Autodesk Inventor part; units mm, degrees
ref_plane "YZ Plane" through (0, 0, 0) normal (1, 0, 0) x (0, 1, 0)
ref_plane "XZ Plane" through (0, 0, 0) normal (0, 1, 0) x (-1, 0, 0)
ref_plane "XY Plane" through (0, 0, 0) normal (0, 0, 1) x (1, 0, 0)
sketch "Эскиз1" plane through (0, 0, 0) normal (0, 1, 0) x (-1, 0, 0)
  line L0 (0, 0) -> (49, 0)
  line L1 (49, 0) -> (49, 43)
  line L2 (49, 43) -> (0, 43)
  line L3 (0, 43) -> (0, 0)
  dimension "d0" = 49
  dimension "d1" = 43
extrude "Выдавливание1" add sketch "Эскиз1" along normal blind 1.5
sketch "Эскиз2" plane through (0, 1.5, 0) normal (0, 1, 0) x (1, 0, 0)
  circle A0 centre (-43.5, -4.7) radius 1.5
  circle A1 centre (-43.5, -38.3) radius 1.5
  circle A2 centre (-5.5, -4.7) radius 1.5
  circle A3 centre (-5.5, -38.3) radius 1.5
  line L0 (-49, 0) -> (-49, -43)
  line L1 (0, 0) -> (-49, 0)
  line L2 (-49, -43) -> (0, -43)
  line L3 (0, -43) -> (0, 0)
  dimension "d4" = 3
  dimension "d5" = 3
  dimension "d6" = 3
  dimension "d7" = 3
  dimension "d8" = 5.5
  dimension "d9" = 5.5
  dimension "d10" = 4.7
  dimension "d11" = 4.7
  dimension "d12" = 5.5
  dimension "d13" = 5.5
  dimension "d14" = 4.7
  dimension "d15" = 4.7
extrude "Выдавливание2" cut sketch "Эскиз2" against normal blind 1.5 contours A0 | A1 | A2 | A3
sketch "Эскиз3" plane through (0, 1.5, 0) normal (0, 1, 0) x (1, 0, 0)
  line L0 (0, 0) -> (-49, 0)
  line L1 (-22.5, 0) -> (-12, 0)
  line L2 (-12, 0) -> (-12, -8)
  line L3 (-12, -8) -> (-22.5, -8)
  line L4 (-22.5, -8) -> (-22.5, 0)
  line L5 (0, -43) -> (0, 0)
  line L6 (-49, -43) -> (0, -43)
  line L7 (-22.5, -43) -> (-12, -43)
  line L8 (-12, -43) -> (-12, -35)
  line L9 (-12, -35) -> (-22.5, -35)
  line L10 (-22.5, -35) -> (-22.5, -43)
  line L11 (0, -33) -> (-8, -33)
  line L12 (-8, -33) -> (-8, -10)
  line L13 (-8, -10) -> (0, -10)
  line L14 (0, -10) -> (0, -33)
  point P0 (0, -10)
  dimension "d18" = 10.5
  dimension "d19" = 8
  dimension "d20" = 12
  dimension "d21" = 8
  dimension "d22" = 8
  dimension "d23" = 10
  dimension "d24" = 10
extrude "Выдавливание3" add sketch "Эскиз3" along normal blind 11
chamfer "Фаска1" distance 3 angle 45 3 edges at (-17.25, 12.5, 8) (-17.25, 12.5, 35) (-8, 12.5, 21.5)
fillet "Сопряжение1" radius 3 4 edges at (0, 0.75, 0) (0, 0.75, 43) (-49, 0.75, 43) (-49, 0.75, 0)
sketch "Эскиз4" plane through (0, 1.5, 0) normal (0, 1, 0) x (1, 0, 0)
  line L0 (-49, -3) -> (-49, -40)
  line L1 (-49, -33) -> (-33, -33)
  line L2 (-33, -33) -> (-33, -10)
  line L3 (-33, -10) -> (-49, -10)
  line L4 (-49, -10) -> (-49, -33)
  line L5 (-22.5, 0) -> (-46, 0)
  line L6 (-46, -43) -> (-22.5, -43)
  point P0 (0, 0)
  dimension "d31" = 23
  dimension "d32" = 16
  dimension "d33" = 43
  dimension "d34" = 10
extrude "Выдавливание4" add sketch "Эскиз4" along normal blind 25
equation "\"d9\" = d8"
equation "\"d11\" = d10"
equation "\"d12\" = d8"
equation "\"d13\" = d12"
equation "\"d14\" = d11"
equation "\"d15\" = d11"
equation "\"d21\" = d19"
properties part number "драйвер"
Source: CAD feature listing. Evaluate the final solid. Frame: model axes, mm. A direction names the side the tool comes from. Give positions to 0.01 mm unless a question says otherwise; leave off trailing zeros. Loops run counter-clockwise (first coordinate to the right, second up) from the corner with the lowest first, then second, coordinate; pieces in that order, holes last. Notation, with made-up numbers: (17, 63.5) -> (36, 63.5) arc R34 cw to (36, 101.5) -> close; hole circle Ø10 at (43, -28.5). An arc over 180 degrees is marked (long way). Put each result on its own line as item: value. Start each with the question number.
1) Contact query for flat-ended pins moving along their axis: P1, Ø1.5, axis at x = -15, z = 1.5, coming from the +Y side; P2, Ø2.5, axis at y = 6, z = 38.5, coming from the -X side; P3, Ø13, axis at x = -43.5, y = 11, coming from the +Z side; P4, Ø10, axis at y = 9, z = 13.5, coming from the +X side. Output: stop coordinate, or through.
2) Cut plane B-B (y = 3.25). Return loops of the section in (x, z), then the cut area to 3 significant figures.
3) Draft query along X for faces 5 (the face through (-48.1, 0.76, 0.86)), 6 (the face through (-12, 7, 39)), 7 (the face through (-6.61, 0.76, 3.69)), 8 (the face through (-20, 5, 43)). Return one class per face: released by +X, released by -X, zero draft, split by the parting line, or undercut.
4) Reachability of faces 1 (the face through (-4, 7, 10)), 2 (the face through (-12, 7, 4)), 3 (the face through (-8, 5, 22)), 4 (the face through (-22.5, 7, 4)) from +Z, -Z, +X, -X, +Y, -Y: full face, straight path, thin tool, end or side. Return the list, or none.
5) Cut plane D-D (z = 12). Return loops of the section in (x, y).
6) Cut plane A-A (x = -43.5). Return loops of the section in (y, z), then the cut area to 4 significant figures.
7) Material intervals for probe 1 along Z at (x, y) = (-5.5, 0.3); probe 2 along X at (y, z) = (1, 38.3); probe 3 along X at (y, z) = (8.75, 23.5), sorted ascending.
8) Cut plane C-C (x = -13). Return loops of the section in (y, z).
Results are:
1. P1: stops at y = 12.5
1. P2: stops at x = -22.5
1. P3: stops at z = 33
1. P4: stops at x = 0
2. outline: (-49, 10) -> (-33, 10) -> (-33, 33) -> (-49, 33) -> close; (-22.5, 0) -> (-12, 0) -> (-12, 8) -> (-22.5, 8) -> close; (-22.5, 35) -> (-12, 35) -> (-12, 43) -> (-22.5, 43) -> close; (-8, 10) -> (0, 10) -> (0, 33) -> (-8, 33) -> close
2. area: 720 mm2
3. face 5: released by -X
3. face 6: released by +X
3. face 7: undercut
3. face 8: zero draft
4. face 1: -Z, +X, -X, +Y
4. face 2: +Z, -Z, +X, +Y
4. face 3: +Z, -Z, +Y
4. face 4: +Z, -Z, -X, +Y
5. outline: (-49, 0) -> (0, 0) -> (0, 12.5) -> (-5, 12.5) -> (-8, 9.5) -> (-8, 1.5) -> (-33, 1.5) -> (-33, 26.5) -> (-49, 26.5) -> close
6. outline: (0, 0) -> (1.5, 0) -> (1.5, 3.2) -> (0, 3.2) -> close; (0, 6.2) -> (1.5, 6.2) -> (1.5, 10) -> (26.5, 10) -> (26.5, 33) -> (1.5, 33) -> (1.5, 36.8) -> (0, 36.8) -> close; (0, 39.8) -> (1.5, 39.8) -> (1.5, 43) -> (0, 43) -> close
6. area: 630.5 mm2
7. probe 1: z = 0 to 3.2, 6.2 to 36.8, 39.8 to 43
7. probe 2: x = -49 to -45, -42 to -7, -4 to 0
7. probe 3: x = -49 to -33, -8 to 0
8. outline: (0, 0) -> (12.5, 0) -> (12.5, 5) -> (9.5, 8) -> (1.5, 8) -> (1.5, 35) -> (9.5, 35) -> (12.5, 38) -> (12.5, 43) -> (0, 43) -> close
